```python
from build123d import *

# Parameters (mm, degrees)
F0_R           = 1.55
F0_R_2         = 14.25
F0_W           = 71.5
F0_H           = 25
F1_DEPTH       = 1.6
F2_W           = 73.9
F2_H           = 27.4
F2_W_2         = 71.5
F2_H_2         = 25
F3_DEPTH       = 1
F5_D           = 3.1
F5_CSINK_D     = 5.5
F5_CSINK_ANGLE = 90


with BuildPart() as f1:
    # F0 (on Top) → F1 (new body)
    with BuildSketch(Plane.XY):
        with BuildLine():
            Line((-42, -94.5), (42, -94.5))
            ThreePointArc((42, -94.5), (44.1213203436, -93.6213203436), (45, -91.5))
            Line((45, -91.5), (45, 24.5))
            ThreePointArc((45, 24.5), (44.1213203436, 26.6213203436), (42, 27.5))
            Line((42, 27.5), (-42, 27.5))
            ThreePointArc((-42, 27.5), (-44.1213203436, 26.6213203436), (-45, 24.5))
            Line((-45, 24.5), (-45, -91.5))
            ThreePointArc((-45, -91.5), (-44.1213203436, -93.6213203436), (-42, -94.5))
        make_face()
        with Locations((-40.5, -90)):
            Circle(F0_R, mode=Mode.SUBTRACT)
        with Locations((-18, -72.5)):
            Circle(F0_R_2, mode=Mode.SUBTRACT)
        with Locations((-18, -36.5)):
            Circle(F0_R_2, mode=Mode.SUBTRACT)
        with Locations((18, -72.5)):
            Circle(F0_R_2, mode=Mode.SUBTRACT)
        with Locations((40.5, -90)):
            Circle(F0_R, mode=Mode.SUBTRACT)
        with Locations((18, -36.5)):
            Circle(F0_R_2, mode=Mode.SUBTRACT)
        with Locations((-40.5, 23)):
            Circle(F0_R, mode=Mode.SUBTRACT)
        Rectangle(F0_W, F0_H, mode=Mode.SUBTRACT)
        with Locations((40.5, 23)):
            Circle(F0_R, mode=Mode.SUBTRACT)
    extrude(amount=F1_DEPTH)

    # F2 (on face) → F3 (join)
    with BuildSketch(Plane.XY.offset(1.6)):
        Rectangle(F2_W, F2_H)
        Rectangle(F2_W_2, F2_H_2, mode=Mode.SUBTRACT)
    extrude(amount=F3_DEPTH)

    # F5 (through all)
    with Locations(Plane.XY.offset(1.6)):
        with Locations((-40.5, 23), (40.5, 23), (-40.5, -90), (40.5, -90)):
            CounterSinkHole(F5_D / 2, F5_CSINK_D / 2, counter_sink_angle=F5_CSINK_ANGLE)


solid = f1.part
```
Can you work these out from the model? Positions are in its coordinate system, mm. A direction names the side the tool comes from. Coordinates: 2 decimals unless noted, no trailing zeros. Loops run counter-clockwise (first coordinate to the right, second up) from the corner with the lowest first, then second, coordinate; pieces in that order, holes last.
Item 1: Suppose I cut it at D-D (y = 2.5). Please give me the cut outline in (x, z), then the cut area to 3 significant figures.
Answers below:
outline: (-45, 0) - (-35.75, 0) - (-35.75, 2.6) - (-36.95, 2.6) - (-36.95, 1.6) - (-45, 1.6) - close; (35.75, 0) - (45, 0) - (45, 1.6) - (36.95, 1.6) - (36.95, 2.6) - (35.75, 2.6) - close
area: 32.0 mm2
Item 2: If we mould it in two halves opening along X, with no side actions, what happens to faces 1 (the face through (-11, -13, 2.6)), 2 (the face through (-11.42, -49.14, 0.79)), 3 (the face through (44.1, -93.64, 0.79)), 4 (the face through (14.91, -86.41, 0.79))? For each: released by +X, released by -X, zero draft, split by the parting line, or undercut.
Answers below:
face 1: zero draft
face 2: undercut
face 3: released by +X
face 4: undercut
Item 3: Which directions (+Z, -Z, +X, -X, +Y, -Y) give clear straight access to the entire face, cutting with the end or side of a thin tool? Please do faces 5 (the face through (-1, 12.5, 1)), 6 (the face through (44.14, 26.6, 0.79)).
Answers below:
face 5: +Z, -Z
face 6: +Z, -Z, +X, +Y
Item 4: Suppose I cut it at B-B (y = 23). Please give me the cut outline in (x, z).
Answers below:
outline: (-45, 0) - (-42.05, 0) - (-42.05, 0.4) - (-43.25, 1.6) - (-45, 1.6) - close; (-38.95, 0) - (38.95, 0) - (38.95, 0.4) - (37.75, 1.6) - (-37.75, 1.6) - (-38.95, 0.4) - close; (42.05, 0) - (45, 0) - (45, 1.6) - (43.25, 1.6) - (42.05, 0.4) - close
Item 5: Please list where these lines run through material, in increasing order: L1, parallel to X at y = -90, z = 0.1; L2, parallel to Y at x = -40.5, z = 0.2; L3, parallel to Y at x = 18, z = 0.6.
Answers below:
L1: x = -45 to -42.05, -38.95 to 38.95, 42.05 to 45
L2: y = -94.5 to -91.55, -88.45 to 21.45, 24.55 to 27.5
L3: y = -94.5 to -86.75, -58.25 to -50.75, -22.25 to -12.5, 12.5 to 27.5
Item 6: Suppose I cut it at C-C (z = 0.9). State how many separate pieces and enclosed holes the cut face has, then the cut area to 3 significant figures.
Answers below:
separate pieces: 1
enclosed holes: 9
area: 6,580 mm2
Item 7: Suppose I cut it at A-A (x = -18). Please give me the cut outline in (y, z), then the cut area to 3 significant figures.
Answers below:
outline: (-94.5, 0) - (-86.75, 0) - (-86.75, 1.6) - (-94.5, 1.6) - close; (-58.25, 0) - (-50.75, 0) - (-50.75, 1.6) - (-58.25, 1.6) - close; (-22.25, 0) - (-12.5, 0) - (-12.5, 2.6) - (-13.7, 2.6) - (-13.7, 1.6) - (-22.25, 1.6) - close; (12.5, 0) - (27.5, 0) - (27.5, 1.6) - (13.7, 1.6) - (13.7, 2.6) - (12.5, 2.6) - close
area: 66.4 mm2
